from build123d import *

# Parameters (mm, degrees)
BOSS_EXTRU_1_DEPTH = 20


with BuildPart() as part:
    # Esquisse1 → Boss.-Extru.1 (new body)
    with BuildSketch(Plane(origin=(0, 0, 0), x_dir=(0, 0, -1), z_dir=(1, 0, 0))):
        with BuildLine():
            Line((5.166852316, 0.172516338), (40, 1.335562371))
            Line((40, 1.335562371), (40, 3.335562371))
            Line((40, 3.335562371), (10, 3.335562371))
            Line((10, 3.335562371), (10, 9.535562371))
            Line((10, 9.535562371), (40, 9.535562371))
            Line((40, 9.535562371), (40, 11.535562371))
            Line((40, 11.535562371), (10, 15))
            Line((10, 15), (10, 23))
            ThreePointArc((10, 23), (9.414213562, 24.414213562), (8, 25))
            Line((8, 25), (6.5, 25))
            Line((6.5, 25), (6.5, 15))
            Line((6.5, 15), (3.5, 15))
            Line((3.5, 15), (3.5, 25))
            Line((3.5, 25), (2, 25))
            ThreePointArc((2, 25), (0.585786438, 24.414213562), (0, 23))
            Line((0, 23), (0, 15))
            Line((0, 15), (0, 5.169731593))
            ThreePointArc((0, 5.169731593), (1.523957824, 1.575690582), (5.166852316, 0.172516338))
        make_face()
    extrude(amount=BOSS_EXTRU_1_DEPTH)


solid = part.part
Design review of the part built by this model. Coordinates are the model's own, in mm. A direction names the side the tool comes from. Give positions to 0.01 mm unless a question says otherwise; leave off trailing zeros. Loops run counter-clockwise (first coordinate to the right, second up) from the corner with the lowest first, then second, coordinate; pieces in that order, holes last. Notation, with made-up numbers: (-32, 23) - (13, 23) arc R4 cw to (13, 27) - close; hole circle Ø4 at (82.25, -15.75). An arc over 180 degrees is marked (long way). Write item = value, one per line.
1) Take a section at D-D on y = 13.25. State the section outline as (x, z) points, and give its area (3 significant figures).
Result sheet:
outline = (0, -25.15) - (20, -25.15) - (20, 0) - (0, 0) - close
area = 503 mm2
2) Draft analysis for pull direction Y (two halves, no side actions). For faces 4 (the face through (10, 2, -40)), 5 (the face through (10, 6, -10)), 6 (the face through (9.86, 24.4, -9.43)), 7 (the face through (10, 3.336, -25)), state which applies: +Y half, -Y half, draft (parallel to the pull), parting line (faces both ways), or undercut.
Result sheet:
face_4 = draft
face_5 = undercut
face_6 = +Y half
face_7 = undercut
3) Clearance check with flat-ended pins moving along their axes: pin 1 Ø4 at (x, y) = (14.5, 19.5) entering from -Z; pin 2 Ø3 at (x, z) = (5, -31.5) entering from -Y; pin 3 Ø6 at (x, z) = (18, -25.5) entering from +Y. State where each tip first meets the part, or that it passes through.
Result sheet:
pin_1 = -10
pin_2 = 1
pin_3 = 13.56
4) Take a section at B-B on y = 21.25. State the section outline as (x, z) points.
Result sheet:
outline = (0, -10) - (20, -10) - (20, -6.5) - (0, -6.5) - close; (0, -3.5) - (20, -3.5) - (20, 0) - (0, 0) - close
5) Take a section at C-C on x = 8.25. State the section outline as (y, z) points.
Result sheet:
outline = (0.17, -5.17) - (1.34, -40) - (3.34, -40) - (3.34, -10) - (9.54, -10) - (9.54, -40) - (11.54, -40) - (15, -10) - (23, -10) arc R2 ccw to (25, -8) - (25, -6.5) - (15, -6.5) - (15, -3.5) - (25, -3.5) - (25, -2) arc R2 ccw to (23, 0) - (5.17, 0) arc R5 ccw to start
6) Take a section at A-A on z = -19. State the section outline as (x, y) points, and give its area (3 significant figures).
Result sheet:
outline = (0, 0.63) - (20, 0.63) - (20, 3.34) - (0, 3.34) - close; (0, 9.54) - (20, 9.54) - (20, 13.96) - (0, 13.96) - close
area = 143 mm2
7) Tool access review of faces 1 (the face through (10, 25, -3)), 2 (the face through (10, 19, -10)), 3 (the face through (10, 20, -3.5)): name each direction out of +Z, -Z, +X, -X, +Y, -Y from which nothing blocks a thin tool from reaching the whole face with its end or side.
Result sheet:
face_1 = +Z, -Z, +X, -X, +Y
face_2 = -Z, +X, -X, +Y
face_3 = +X, -X, +Y
8) To check wall thickness, follow line 1 (Z direction, x = 18.5, y = 15.5); line 2 (Y direction, x = 5.75, z = -34.5); line 3 (Y direction, x = 4, z = -21). State the ranges of each line that lie inside material, in increasing order.
Result sheet:
line_1 = -10 to -6.5, -3.5 to 0
line_2 = 1.15 to 3.34, 9.54 to 12.17
line_3 = 0.7 to 3.34, 9.54 to 13.73
